Geometry check sheet. Reference: the model listing, model coordinates, mm. Face numbers are marked on the shaded views. A direction names the side the tool comes from. Round coordinates to 2 decimals unless told otherwise and drop trailing zeros. Write each loop counter-clockwise with the first axis right and the second up, starting at its lowest first coordinate (ties: lowest second). Pieces come first, ordered by that corner, then holes. Notation, with made-up numbers: (88, -11.75) -> (145, -11.75) arc R7 cw to (145, -3.75) -> close; hole circle Ø6 at (-2, -15.75). An arc over 180 degrees is marked (long way). Use a Markdown table: item, result.
```python
from build123d import *

# Parameters (mm, degrees)
BOSS_EXTRUDE1_DEPTH     = 20
CUT_EXTRUDE1_DEPTH      = 9
CUT_EXTRUDE1_DEPTH_BACK = 9
SKETCH8_R               = 1.55
SKETCH11_R              = 6
BOSS_EXTRUDE12_DEPTH    = 22
SKETCH12_R              = 4
BOSS_EXTRUDE13_DEPTH    = 8
BOSS_EXTRUDE14_DEPTH    = 7
SKETCH14_R              = 1.55
CUT_EXTRUDE2_DEPTH      = 6.1
SKETCH15_R              = 3
BOSS_EXTRUDE15_DEPTH    = 10
CUT_EXTRUDE5_START      = 9
SKETCH16_R              = 3.5
CUT_EXTRUDE5_DEPTH      = 3
CUT_EXTRUDE6_START      = -6
SKETCH16_2_R            = 3.5
CUT_EXTRUDE6_DEPTH      = 3
SKETCH17_R              = 1.55
CUT_EXTRUDE7_DEPTH      = 3


with BuildPart() as part:
    # Sketch1 → Boss-Extrude1 (new body)
    with BuildSketch(Plane.XY):
        with BuildLine():
            Line((-8.708203932, 12), (8.708203932, 12))
            Line((8.708203932, 12), (8.708203932, 9))
            Line((8.708203932, 9), (2.708203932, 9))
            Line((2.708203932, 9), (2.708203932, 6))
            Line((2.708203932, 6), (6.708203932, 6))
            ThreePointArc((6.708203932, 6), (0, -9), (-6.708203932, 6))
            Line((-6.708203932, 6), (-2.708203932, 6))
            Line((-2.708203932, 6), (-2.708203932, 9))
            Line((-2.708203932, 9), (-8.708203932, 9))
            Line((-8.708203932, 9), (-8.708203932, 12))
        make_face()
        Polygon((0, 4.4), (-3.810511777, 2.2), (-3.810511777, -2.2), (0, -4.4), (3.810511777, -2.2), (3.810511777, 2.2), align=None, mode=Mode.SUBTRACT)
    extrude(amount=BOSS_EXTRUDE1_DEPTH)

    # Sketch8 → Cut-Extrude1 (cut, two sides: drawn at the far end of the back side and taken through both)
    with BuildSketch(Plane.ZY.offset(-CUT_EXTRUDE1_DEPTH_BACK)):
        with Locations(Location((6, 0, 0), (0, 0, 180))):
            Circle(SKETCH8_R)
        with Locations(Location((14, 0, 0), (0, 0, 180))):
            Circle(SKETCH8_R)
    extrude(amount=CUT_EXTRUDE1_DEPTH + CUT_EXTRUDE1_DEPTH_BACK, mode=Mode.SUBTRACT)

    # Sketch11 → Boss-Extrude12 (add)
    with BuildSketch(Plane(origin=(0, 0, 0), x_dir=(-1, 0, 0), z_dir=(0, 0, -1))):
        with Locations(Location((0, 0, 0), (0, 0, 180))):
            Circle(SKETCH11_R)
    extrude(amount=BOSS_EXTRUDE12_DEPTH)

    # Sketch12 → Boss-Extrude13 (add)
    with BuildSketch(Plane(origin=(0, 0, -22), x_dir=(-1, 0, 0), z_dir=(0, 0, -1))):
        Circle(SKETCH12_R)
    extrude(amount=BOSS_EXTRUDE13_DEPTH)

    # Sketch13 → Boss-Extrude14 (add)
    with BuildSketch(Plane(origin=(0, 0, -30), x_dir=(-1, 0, 0), z_dir=(0, 0, -1))):
        Polygon((1.75, 3.031088913), (-1.75, 3.031088913), (-3.5, 0), (-1.75, -3.031088913), (1.75, -3.031088913), (3.5, 0), align=None)
    extrude(amount=BOSS_EXTRUDE14_DEPTH)

    # Sketch14 → Cut-Extrude2 (cut)
    with BuildSketch(Plane(origin=(2.625, -1.515544457, 0), x_dir=(0, 0, -1), z_dir=(0.8660254037844379, -0.5000000000000011, 0))):
        with Locations(Location((33.5, 0, 0), (0, 0, 90))):
            Circle(SKETCH14_R)
    extrude(amount=-CUT_EXTRUDE2_DEPTH, mode=Mode.SUBTRACT)

    # Sketch15 → Boss-Extrude15 (add)
    with BuildSketch(Plane(origin=(0, 0, -37), x_dir=(-1, 0, 0), z_dir=(0, 0, -1))):
        Circle(SKETCH15_R)
    extrude(amount=BOSS_EXTRUDE15_DEPTH)

    # Sketch16 → Cut-Extrude5 (cut)
    with BuildSketch(Plane.ZY.offset(CUT_EXTRUDE5_START)):
        with Locations((6, 0)):
            Circle(SKETCH16_R)
        with Locations((14, 0)):
            Circle(SKETCH16_R)
    extrude(amount=-CUT_EXTRUDE5_DEPTH, mode=Mode.SUBTRACT)

    # Sketch16<2> → Cut-Extrude6 (cut)
    with BuildSketch(Plane.ZY.offset(CUT_EXTRUDE6_START)):
        with Locations((6, 0)):
            Circle(SKETCH16_2_R)
        with Locations((14, 0)):
            Circle(SKETCH16_2_R)
    extrude(amount=-CUT_EXTRUDE6_DEPTH, mode=Mode.SUBTRACT)

    # Sketch17 → Cut-Extrude7 (cut)
    with BuildSketch(Plane(origin=(0, 12, 0), x_dir=(1, 0, 0), z_dir=(0, 1, 0))):
        with Locations(Location((-4.242640687, -5.757359313, 0), (0, 0, 270))):
            Circle(SKETCH17_R)
        with Locations(Location((4.242640687, -5.757359313, 0), (0, 0, 270))):
            Circle(SKETCH17_R)
        with Locations(Location((4.242640687, -14.242640687, 0), (0, 0, 270))):
            Circle(SKETCH17_R)
        with Locations(Location((-4.242640687, -14.242640687, 0), (0, 0, 270))):
            Circle(SKETCH17_R)
    extrude(amount=-CUT_EXTRUDE7_DEPTH, mode=Mode.SUBTRACT)


solid = part.part
```
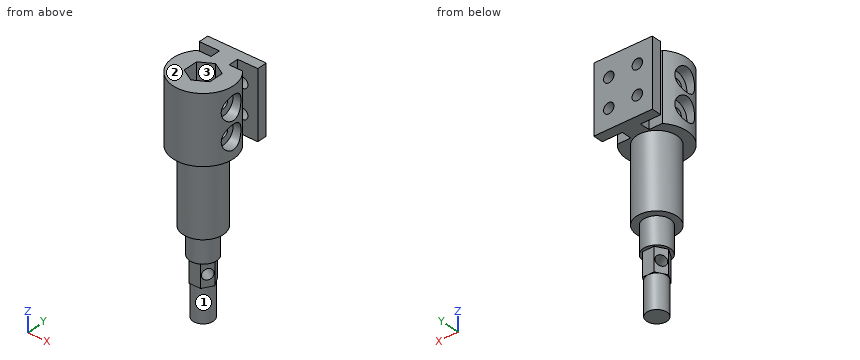
(1) Section check C-C on y = -5. Record the cut outline in (x, z), plus the area to 3 significant figures.
A:
| item | result |
|---|---|
| outline | (-7.48, 0) -> (-3.32, 0) -> (-3.32, -22) -> (3.32, -22) -> (3.32, 0) -> (7.48, 0) -> (7.48, 20) -> (-7.48, 20) -> close |
| area | 445 mm2 |
(2) Thickness scan on line 1 (Y direction, x = -6.25, z = 5); line 2 (Y direction, x = -7.9, z = 6); line 3 (Z direction, x = -0.75, y = 0.25). Record the ranges inside material, lowest first.
A:
| item | result |
|---|---|
| line 1 | y = -6.48 to -3.35, 3.35 to 6, 9 to 12 |
| line 2 | y = -4.31 to -3.5, 3.5 to 4.31, 9 to 12 |
| line 3 | z = -47 to -35.04, -31.96 to 0 |
(3) Gauge pin test, flat ends, axial feed: pin 1 Ø3 at (x, z) = (5, 5.5) entering from -Y; pin 2 Ø2.5 at (x, z) = (4.24, 14.24) entering from -Y; pin 3 Ø6.5 at (y, z) = (0, 6) entering from +X. Record the tip position at first contact, or that the pin passes through.
A:
| item | result |
|---|---|
| pin 1 | stops at y = -8.29 |
| pin 2 | stops at y = -8.49 |
| pin 3 | stops at x = 6 |
(4) Access from +Z, -Z, +X, -X, +Y, -Y to the whole of each face (thin tool, end or side, straight path). Record for the marked faces 1, 2 and 3.
A:
| item | result |
|---|---|
| face 1 | -Z |
| face 2 | +Z, +X, -X, +Y, -Y |
| face 3 | +Z |
(5) Section check B-B on z = -9.5. Record the cut outline in (x, y), plus the area to 3 significant figures.
A:
| item | result |
|---|---|
| outline | circle Ø12 at (0, 0) |
| area | 113 mm2 |
(6) Section check A-A on y = 6.75. Record the cut outline in (x, z), plus the area to 3 significant figures.
A:
| item | result |
|---|---|
| outline | (-2.71, 0) -> (2.71, 0) -> (2.71, 20) -> (-2.71, 20) -> close |
| area | 108 mm2 |
